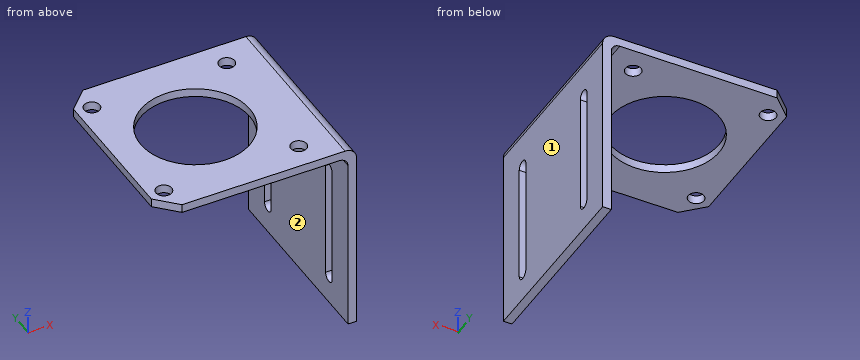
Autodesk Inventor part; units mm, degrees
ref_plane "YZ Plane" through (0, 0, 0) normal (1, 0, 0) x (0, 1, 0)
ref_plane "XZ Plane" through (0, 0, 0) normal (0, 1, 0) x (-1, 0, 0)
ref_plane "XY Plane" through (0, 0, 0) normal (0, 0, 1) x (1, 0, 0)
sketch "Sketch1" plane through (0, 0, 0) normal (0, 1, 0) x (-1, 0, 0)
  line L0 (4, 0) -> (68, 0)
  line L1 (0, -4) -> (0, -68)
  line L2 (68, -3) -> (6, -3)
  line L3 (3, -6) -> (3, -68)
  line L4 (68, 0) -> (68, -3)
  line L5 (3, -68) -> (0, -68)
  arc A0 (4, 0) -> (0, -4) centre (4, -4) ccw
  arc A1 (6, -3) -> (3, -6) centre (6, -6) ccw
  point P0 (0, 0)
  dimension "d0" = 68
  dimension "d1" = 68
  dimension "d2" = 3
  dimension "d3" = 4
  dimension "d4" = 3
extrude "Extrusion1" add sketch "Sketch1" along normal blind 65
sketch "Sketch2" plane through (-68, 0, 0) normal (0, 0, 1) x (1, 0, 0)
  circle A0 centre (29, 32.5) radius 19.05
  point P0 (68, 0)
  point P1 (0, 65)
  dimension "d8" = 38.1
extrude "Extrusion2" cut sketch "Sketch2" against normal blind 3
sketch "Sketch3" plane through (-68, 0, 0) normal (0, 0, 1) x (1, 0, 0)
  circle A0 centre (5.43, 8.93) radius 2.75
  point P0 (68, 0)
  dimension "d13" = 5.5
extrude "Extrusion3" cut sketch "Sketch3" against normal blind 3
pattern_linear "Rectangular Pattern1" count 2 spacing 47.14 along (0, 1, 0) count 2 spacing 47.14 along (1, 0, 0) of "Extrusion3"
sketch "Sketch4" plane through (0, 0, -4) normal (1, 0, 0) x (0, 0, -1)
  arc A0 (53.8, 50.35) -> (53.8, 54.65) centre (53.8, 52.5) ccw
  arc A1 (12.1, 54.65) -> (12.1, 50.35) centre (12.1, 52.5) ccw
  line L0 (53.8, 54.65) -> (12.1, 54.65)
  line L1 (53.8, 50.35) -> (12.1, 50.35)
  line L2 (46.8257, 32.5) -> (19.3775, 32.5)
  arc A2 (53.8, 10.35) -> (53.8, 14.65) centre (53.8, 12.5) ccw
  arc A3 (12.1, 14.65) -> (12.1, 10.35) centre (12.1, 12.5) ccw
  line L3 (53.8, 10.35) -> (12.1, 10.35)
  line L4 (53.8, 14.65) -> (12.1, 14.65)
  point P0 (-4, 0)
  dimension "d24" = 4.3
  dimension "d26" = 4.3
extrude "Extrusion4" cut sketch "Sketch4" against normal blind 3
chamfer "Chamfer1" distance 7 angle 45 2 edges at (-68, 65, -1.5) (-68, 0, -1.5)
properties part number "Soporte Motor"
Can you work these out from the model? Positions are in its coordinate system, mm. Face numbers are marked on the shaded views. A direction names the side the tool comes from. Give positions to 0.01 mm unless a question says otherwise; leave off trailing zeros. Order: outer loops, then holes, each group sorted by start corner. A loop starts at its lowest first (then second) coordinate and runs counter-clockwise, first axis right, second up. Notation, with made-up numbers: M -24,53.5 L 10,53.5 A14 ccw 10,77.5 Z; hole C 69,13 d7. An arc over 180 degrees is marked long. One line per item, written item: value.
1) Please list where these lines run through material, in increasing order: line 1 along Y through (x, z) = (-15.43, -1.7); line 2 along Y through (x, z) = (-62, -1); line 3 along Y through (x, z) = (-39, -1).
Answer sheet:
line 1: y = 0 to 6.18, 11.68 to 53.32, 58.82 to 65
line 2: y = 1 to 6.24, 11.62 to 53.38, 58.76 to 64
line 3: y = 0 to 13.45, 51.55 to 65
2) I want a section at C-C, the plane x = -15.43. List the corners of the cut face in (y, z) for me.
Answer sheet:
outline: M 0,-3 L 6.18,-3 L 6.18,0 L 0,0 Z; M 11.68,-3 L 53.32,-3 L 53.32,0 L 11.68,0 Z; M 58.82,-3 L 65,-3 L 65,0 L 58.82,0 Z
3) For P1, Ø2, axis at x = -29.5, y = 17, coming from the -Z side; P2, Ø9, axis at x = -62.57, y = 8.93, coming from the +Z side; P3, Ø2, axis at y = 50.5, z = -34, coming from the -X side, each with a flat end and sliding along its axis, tell me the tip position at first contact or that it passes through.
Answer sheet:
P1: stops at z = -3
P2: stops at z = 0
P3: stops at x = -3
4) I want a section at D-D, the plane y = 47. List the corners of the cut face in (x, z) for me, plus the area to 3 significant figures.
Answer sheet:
outline: M -68,-3 L -51.36,-3 L -51.36,0 L -68,0 Z; M -26.64,-3 L -6,-3 A3 cw -3,-6 L -3,-68 L 0,-68 L 0,-4 A4 ccw -4,0 L -26.64,0 Z
area: 323 mm^2
5) On a 3-axis mill with a long thin cutter (end or side, diameter ignored), from which of +Z, -Z, +X, -X, +Y, -Y can I reach the whole of each face in a straight line? I mean the marked faces 1 and 2. Say none if no direction works.
Answer sheet:
face 1: +Z, -Z, +X, +Y, -Y
face 2: -Z, -X, +Y, -Y
6) I want a section at B-B, the plane z = -29. List the corners of the cut face in (x, y) for me.
Answer sheet:
outline: M -3,0 L 0,0 L 0,10.35 L -3,10.35 Z; M -3,14.65 L 0,14.65 L 0,50.35 L -3,50.35 Z; M -3,54.65 L 0,54.65 L 0,65 L -3,65 Z
7) I want a section at A-A, the plane y = 56.07. List the corners of the cut face in (x, z) for me, plus the area to 3 significant figures.
Answer sheet:
outline: M -68,-3 L -65.32,-3 L -65.32,0 L -68,0 Z; M -59.82,-3 L -18.18,-3 L -18.18,0 L -59.82,0 Z; M -12.68,-3 L -6,-3 A3 cw -3,-6 L -3,-68 L 0,-68 L 0,-4 A4 ccw -4,0 L -12.68,0 Z
area: 364 mm^2
